from build123d import *

# Parameters (mm, degrees)
SKETCH2_R           = 20
SKETCH2_R_2         = 2
BOSS_EXTRUDE1_DEPTH = 4
FILLET2_SIZE        = 2


with BuildPart() as part:
    # Sketch2 → Boss-Extrude1 (new body)
    with BuildSketch(Plane(origin=(0, 0, 0), x_dir=(1, 0, 0), z_dir=(0, 1, 0))):
        with Locations(Location((0, 0, 0), (0, 0, 270))):
            Circle(SKETCH2_R)
        with BuildLine():
            Line((-2.5, 14.790199458), (-2.5, 2.5))
            Line((-2.5, 2.5), (-14.790199458, 2.5))
            ThreePointArc((-14.790199458, 2.5), (-10.606601718, 10.606601718), (-2.5, 14.790199458))
        make_face(mode=Mode.SUBTRACT)
        with BuildLine():
            Line((-14.790199458, -2.5), (-2.5, -2.5))
            Line((-2.5, -2.5), (-2.5, -14.790199458))
            ThreePointArc((-2.5, -14.790199458), (-10.606601718, -10.606601718), (-14.790199458, -2.5))
        make_face(mode=Mode.SUBTRACT)
        with BuildLine():
            Line((2.5, -14.790199458), (2.5, -2.5))
            Line((2.5, -2.5), (14.790199458, -2.5))
            ThreePointArc((14.790199458, -2.5), (10.606601718, -10.606601718), (2.5, -14.790199458))
        make_face(mode=Mode.SUBTRACT)
        with BuildLine():
            Line((14.790199458, 2.5), (2.5, 2.5))
            Line((2.5, 2.5), (2.5, 14.790199458))
            ThreePointArc((2.5, 14.790199458), (10.606601718, 10.606601718), (14.790199458, 2.5))
        make_face(mode=Mode.SUBTRACT)
        with Locations(Location((0, 0, 0), (0, 0, 270))):
            Circle(SKETCH2_R_2, mode=Mode.SUBTRACT)
    extrude(amount=BOSS_EXTRUDE1_DEPTH)

    # Fillet2
    # a fillet whose section is not a circle: 2 mm, written as the material it takes off along each edge
    with BuildSketch(Plane(origin=(0, 4, 0), x_dir=(0, 0, 1), z_dir=(-1, 0, 0))) as fillet2_piece_1:
        with BuildLine():
            Bezier((20, -FILLET2_SIZE), (20, 0), (20 - FILLET2_SIZE, 0), weights=[1, 0.471404521, 1])
            Line((20 - FILLET2_SIZE, 0), (20, 0))
            Line((20, 0), (20, -FILLET2_SIZE))
        make_face()
    revolve(axis=Axis((0, 4, 0), (0, 1, 0)), mode=Mode.SUBTRACT)


solid = part.part
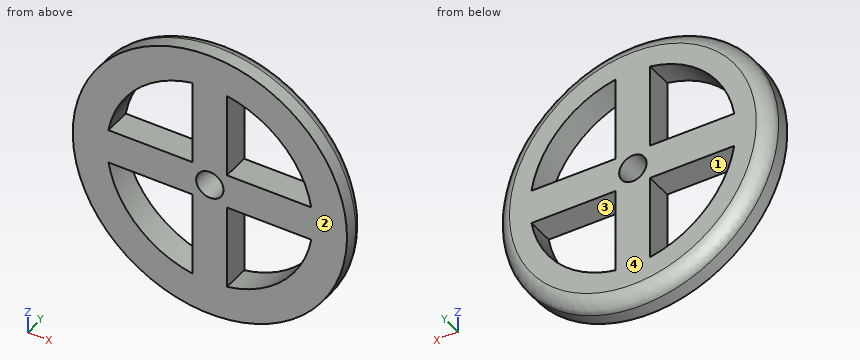
Can you work these out from the model? Positions are in its coordinate system, mm. Face numbers are marked on the shaded views. A direction names the side the tool comes from. Coordinates: 2 decimals unless noted, no trailing zeros. Return JSON: item names as keys, results as strings. Group by question number.
Item 1: Please list where these lines run through material, in increasing order: probe 1 along X at (y, z) = (1.85, 0); probe 2 along X at (y, z) = (2.3, -3); probe 3 along X at (y, z) = (1.25, -11.5).
Item 2: Which directions (+Z, -Z, +X, -X, +Y, -Y) give clear straight access to the entire face, cutting with the end or side of a thin tool? Please do the marked faces 1 and 2.
Item 3: I'm going to push flat-ended pins straight in: pin 1 Ø1.2 at (x, y) = (-6, 1) entering from +Z; pin 2 Ø1.2 at (x, y) = (-7.5, 2.5) entering from -Z; pin 3 Ø1 at (y, z) = (3, 5.5) entering from -X; pin 4 Ø3.5 at (x, z) = (0, 0) entering from -Y. Where does each tip first touch, or does it pass through?
Item 4: We'd pull the mould along Z, two halves only. Please class the marked faces 3 and 4: pulls with the +Z half, pulls with the -Z half, needs draft (parallel to the pull), parting line crosses it, or undercut.
Item 5: If we section it at A-A (x = -4): Count the separate pieces of the cut face and the enclosed holes in it, then the cut area to 3 significant figures.
Return value:
{
 "1": {"probe 1": "x = -20 to -2, 2 to 20", "probe 2": "x = -19.73 to -14.7, -2.5 to 2.5, 14.7 to 19.73", "probe 3": "x = -16.36 to -9.63, -2.5 to 2.5, 9.63 to 16.36"},
 "2": {"face 1": "+Y, -Y", "face 2": "+Z, -Z, +X, -X, -Y"},
 "3": {"pin 1": "stops at z = 19.26", "pin 2": "stops at z = -18.72", "pin 3": "stops at x = -19.15", "pin 4": "passes through"},
 "4": {"face 3": "undercut", "face 4": "needs draft"},
 "5": {"separate pieces": "3", "enclosed holes": "0", "area": "58.9 mm^2"}
}
